Can you work these out from the model? Positions are in its coordinate system, mm. Face numbers are marked on the shaded views. Round coordinates to 2 decimals unless told otherwise and drop trailing zeros. Order: outer loops, then holes, each group sorted by start corner. A loop starts at its lowest first (then second) coordinate and runs counter-clockwise, first axis right, second up.
Q1. Will these pins go through, and if not, where does the flat tip stop? P1, Ø1.5, axis at x = 13, y = 5, coming from the +Z side; P2, Ø2, axis at x = -8, y = 10.5, coming from the -Z side; P3, Ø1, axis at y = 7.5, z = 1, coming from the +X side.
Q2. We'd pull the mould along Z, two halves only. Please class the marked faces 1, 2 and 3: pulls with the +Z half, pulls with the -Z half, needs draft (parallel to the pull), parting line crosses it, or undercut.
Q3. If I drill on line 1 (X direction, y = 31.3, z = 0); line 2 (X direction, y = 15.25, z = 0); line 3 (Z direction, x = 14, y = 31.5), over which ranges is the centre line in solid material (lowest first)?
Q4. If we section it at B-B (z = 0): Please give me the cut outline in (x, y).
Q5. If we section it at A-A (x = 0): Please give me the cut outline in (y, z).
Q6. If we section it at C-C (y = 3): Please give me the cut outline in (x, z).
from build123d import *

# Parameters (mm, degrees)
SKETCH1_R           = 19
BOSS_EXTRUDE1_DEPTH = 33
SKETCH2_R           = 16
CUT_EXTRUDE1_DEPTH  = 5
SKETCH3_R           = 17.5
CUT_EXTRUDE2_DEPTH  = 28


with BuildPart() as part:
    # Sketch1 → Boss-Extrude1 (new body)
    with BuildSketch(Plane(origin=(0, 0, 0), x_dir=(1, 0, 0), z_dir=(0, 1, 0))):
        with Locations(Location((0, 0, 0), (0, 0, 270))):
            Circle(SKETCH1_R)
    extrude(amount=BOSS_EXTRUDE1_DEPTH)

    # Sketch2 → Cut-Extrude1 (cut)
    with BuildSketch(Plane(origin=(0, 33, 0), x_dir=(1, 0, 0), z_dir=(0, 1, 0))):
        with Locations(Location((0, 0, 0), (0, 0, 270))):
            Circle(SKETCH2_R)
    extrude(amount=-CUT_EXTRUDE1_DEPTH, mode=Mode.SUBTRACT)

    # Sketch3 → Cut-Extrude2 (cut)
    with BuildSketch(Plane.XZ):
        with Locations(Location((0, 0, 0), (0, 0, 270))):
            Circle(SKETCH3_R)
    extrude(amount=-CUT_EXTRUDE2_DEPTH, mode=Mode.SUBTRACT)


solid = part.part
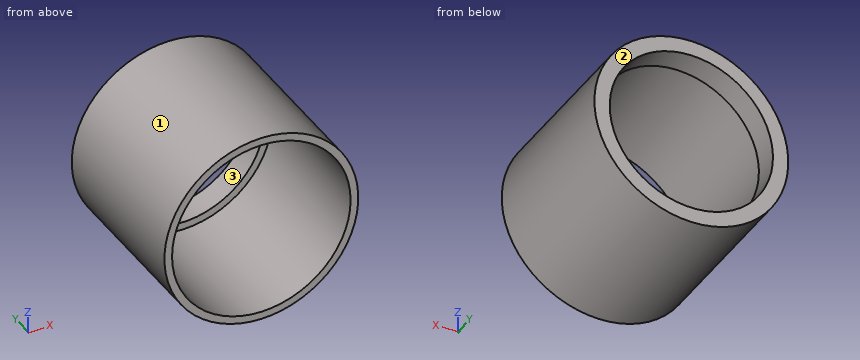
Solution:
1. P1: stops at z = 14.52
1. P2: stops at z = -17.66
1. P3: stops at x = 18.99
2. face 1: parting line crosses it
2. face 2: needs draft
2. face 3: undercut
3. line 1: x = -19 to -16, 16 to 19
3. line 2: x = -19 to -17.5, 17.5 to 19
3. line 3: z = -12.85 to -7.75, 7.75 to 12.85
4. outline: (-19, 0) - (-17.5, 0) - (-17.5, 28) - (-16, 28) - (-16, 33) - (-19, 33) - close; (16, 28) - (17.5, 28) - (17.5, 0) - (19, 0) - (19, 33) - (16, 33) - close
5. outline: (0, -19) - (33, -19) - (33, -16) - (28, -16) - (28, -17.5) - (0, -17.5) - close; (0, 17.5) - (28, 17.5) - (28, 16) - (33, 16) - (33, 19) - (0, 19) - close
6. outline: circle Ø38 at (0, 0); hole circle Ø35 at (0, 0)
